from build123d import *

# Parameters (mm, degrees)
BOSS_EXTRUDE1_DEPTH      = 1040
BOSS_EXTRUDE1_DEPTH_BACK = 360
SKETCH2_R                = 7.5
BOSS_EXTRUDE2_DEPTH      = 680
SKETCH4_W                = 580
SKETCH4_H                = 10
CUT_EXTRUDE1_DEPTH       = 1252.319303775
CUT_EXTRUDE2_DEPTH       = 1252.319303775
CUT_EXTRUDE2_DEPTH_BACK  = 1252.319303775
SKETCH5_W                = 580
SKETCH5_H                = 50
CUT_EXTRUDE3_DEPTH       = 1252.319303775
CUT_EXTRUDE3_DEPTH_BACK  = 1252.319303775
SKETCH6_R                = 7.5
SKETCH8_W                = 25
SKETCH8_H                = 32
BOSS_EXTRUDE4_DEPTH      = 37.5
SKETCH9_W                = 16.002
SKETCH9_H                = 32.5
CUT_EXTRUDE4_DEPTH       = 66.8
SKETCH11_W               = 16.002
SKETCH11_H               = 64
CUT_EXTRUDE5_DEPTH       = 24
SKETCH13_R               = 2.5908
CUT_EXTRUDE6_DEPTH       = 20


with BuildPart() as part:
    # Sketch1 → Boss-Extrude1 (new, two sides: drawn at the far end of the back side and taken through both)
    with BuildSketch(Plane.XY.offset(-BOSS_EXTRUDE1_DEPTH_BACK)):
        with BuildLine():
            Line((0, 0), (-598.236730193, 0))
            ThreePointArc((-598.236730193, 0), (-599.97321197, 0.15192247), (-601.656931626, 0.603073792))
            Line((-601.656931626, 0.603073792), (-690, 32.757321084))
            Line((-690, 32.757321084), (-690, -30))
            Line((-690, -30), (-656.445665216, -30))
            Line((-656.445665216, -30), (-26.446144718, -30))
            Line((-26.446144718, -30), (0, -30))
            Line((0, -30), (0, -20.000479502))
            Line((0, -20.000479502), (0, 0))
        make_face()
    extrude(amount=BOSS_EXTRUDE1_DEPTH + BOSS_EXTRUDE1_DEPTH_BACK)

    # Sketch2 → Boss-Extrude2 (add)
    # profile 1 of 2: a face of its own
    with BuildSketch(Plane.XY):
        with BuildLine():
            Line((-690, -30), (-690, -80))
            ThreePointArc((-690, -80), (-687.071067812, -87.071067812), (-680, -90))
            Line((-680, -90), (-350, -90))
            ThreePointArc((-350, -90), (-342.928932188, -87.071067812), (-340, -80))
            Line((-340, -80), (-340, -30))
            Line((-340, -30), (-690, -30))
        make_face()
        with BuildLine():
            Line((-677.5, -72.5), (-352.5, -72.5))
            ThreePointArc((-352.5, -72.5), (-345, -80), (-352.5, -87.5))
            Line((-352.5, -87.5), (-677.5, -87.5))
            ThreePointArc((-677.5, -87.5), (-685, -80), (-677.5, -72.5))
        make_face(mode=Mode.SUBTRACT)
    # profile 2 of 2: a face of its own
    with BuildSketch(Plane.XY):
        with BuildLine():
            Line((-15, -30), (-15, -80))
            ThreePointArc((-15, -80), (-17.928932188, -87.071067812), (-25, -90))
            Line((-25, -90), (-30, -90))
            ThreePointArc((-30, -90), (-37.071067812, -87.071067812), (-40, -80))
            Line((-40, -80), (-40, -30))
            Line((-40, -30), (-15, -30))
        make_face()
        with Locations((-27.5, -80)):
            Circle(SKETCH2_R, mode=Mode.SUBTRACT)
    extrude(amount=BOSS_EXTRUDE2_DEPTH)

    # Sketch4 → Cut-Extrude1 (cut, through all)
    with BuildSketch(Plane(origin=(0, 0, 0), x_dir=(0, 0, -1), z_dir=(1, 0, 0))):
        with Locations((-340, -85)):
            Rectangle(SKETCH4_W, SKETCH4_H)
    extrude(amount=-CUT_EXTRUDE1_DEPTH, mode=Mode.SUBTRACT)

    # Sketch5 → Cut-Extrude2 (cut, two sides: drawn at the far end of the back side and taken through both)
    with BuildSketch(Plane.ZY.offset(690).offset(-CUT_EXTRUDE2_DEPTH_BACK)):
        with Locations((340, -55)):
            Rectangle(SKETCH5_W, SKETCH5_H)
    extrude(amount=CUT_EXTRUDE2_DEPTH + CUT_EXTRUDE2_DEPTH_BACK, mode=Mode.SUBTRACT)

    # Sketch6 → Cut-Extrude3 (cut, two sides: drawn at the far end of the back side and taken through both)
    with BuildSketch(Plane(origin=(0, 0, 0), x_dir=(1, 0, 0), z_dir=(0, 1, 0)).offset(-CUT_EXTRUDE3_DEPTH_BACK)):
        with Locations((-298.236730193, 60)):
            Circle(SKETCH6_R)
    extrude(amount=CUT_EXTRUDE3_DEPTH + CUT_EXTRUDE3_DEPTH_BACK, mode=Mode.SUBTRACT)

    # Sketch8 → Boss-Extrude4 (add)
    with BuildSketch(Plane.XZ.offset(30)):
        with Locations((-298.236730193, -60)):
            Rectangle(SKETCH8_W, SKETCH8_H)
    extrude(amount=BOSS_EXTRUDE4_DEPTH)

    # Sketch9 → Cut-Extrude4 (cut)
    with BuildSketch(Plane.XY.offset(-44)):
        with Locations((-298.237730193, -46.25)):
            Rectangle(SKETCH9_W, SKETCH9_H)
    extrude(amount=-CUT_EXTRUDE4_DEPTH, mode=Mode.SUBTRACT)

    # Sketch11 → Cut-Extrude5 (cut)
    with BuildSketch(Plane.XZ.offset(30)):
        with Locations((-298.237730193, -60)):
            Rectangle(SKETCH11_W, SKETCH11_H)
    extrude(amount=-CUT_EXTRUDE5_DEPTH, mode=Mode.SUBTRACT)

    # Sketch13 → Cut-Extrude6 (cut)
    with BuildSketch(Plane(origin=(0, 0, 0), x_dir=(1, 0, 0), z_dir=(0, 1, 0))):
        with Locations(Location((-300, -1015, 0), (0, 0, 180))):
            Circle(SKETCH13_R)
        with Locations(Location((-287.3, -360.9, 0), (0, 0, 180))):
            Circle(SKETCH13_R)
        with Locations(Location((-312.7, -360.9, 0), (0, 0, 180))):
            Circle(SKETCH13_R)
    extrude(amount=-CUT_EXTRUDE6_DEPTH, mode=Mode.SUBTRACT)


solid = part.part
Source: CAD feature listing. Evaluate the final solid. Frame: model axes, mm. A direction names the side the tool comes from. Round coordinates to 2 decimals unless told otherwise and drop trailing zeros. Loops run counter-clockwise (first coordinate to the right, second up) from the corner with the lowest first, then second, coordinate; pieces in that order, holes last. Notation, with made-up numbers: M 66.25,86.25 L 72.25,86.25 A16 ccw 72.25,114.25 Z; hole C 33,31 d10. An arc over 180 degrees is marked long. Return JSON: item names as keys, results as strings. Group by question number.
1. Reachability of faces 4 (the face through (-27, -53, 0)), 5 (the face through (-27, -60, 630)), 6 (the face through (-290, -48, -44)), 7 (the face through (-340, -55, 25)), 8 (the face through (-306.239, -28, -60)) from +Z, -Z, +X, -X, +Y, -Y: full face, straight path, thin tool, end or side. Return the list, or none.
2. Mould query, pull axis X, two halves, no side actions, for faces 1 (the face through (-295, 0, 330)), 2 (the face through (-513, -87.5, 655)), 3 (the face through (-285.737, -48, -60)). Classes: released by +X, released by -X, zero draft, split by the parting line, or undercut.
3. Material intervals for line 1 along X through (y, z) = (-4.5, 360.9); line 2 along Z through (x, y) = (-300, -15); line 3 along X through (y, z) = (-80, 13), sorted ascending. Write a range as from..to.
4. Section query B-B on z = 662. Output: boundary loops of the cut face in (x, y), and give its area (3 significant figures).
5. Pin query (flat end, axial travel): pin 1 (5 mm diameter, centred on x = -111.5, z = 163, fed in from -Y); pin 2 (7.5 mm diameter, centred on x = -26, y = -56.5, fed in from -Z); pin 3 (25 mm diameter, centred on x = -552, z = 663, fed in from +Y). Return the tip coordinate at first contact, or that it passes through.
6. Section query C-C on x = -441. Output: boundary loops of the cut face in (y, z).
7. Section query D-D on z = 480. Output: boundary loops of the cut face in (x, y).
8. Section query A-A on y = -46.5. Output: boundary loops of the cut face in (x, z), and give its area (3 significant figures).
Checks:
{
 "1": {"face 4": "-Z, +X, -X, -Y", "face 5": "+X, -X, -Y", "face 6": "+Z, +X, -X, -Y", "face 7": "+Z, -Z, -Y", "face 8": "none"},
 "2": {"face 1": "zero draft", "face 2": "undercut", "face 3": "released by +X"},
 "3": {"line 1": "x = -690..-315.29, -310.11..-289.89, -284.71..0", "line 2": "z = -360..-92, -28..1012.41, 1017.59..1040", "line 3": "x = -690..-685, -345..-340, -40..-35, -20..-15"},
 "4": {"outline": "M -690,-80 A10 ccw -680,-90 L -350,-90 A10 ccw -340,-80 L -340,-30 L -40,-30 L -40,-80 A10 ccw -30,-90 L -25,-90 A10 ccw -15,-80 L -15,-30 L 0,-30 L 0,0 L -598.24,0 A10 cw -601.66,0.6 L -690,32.76 Z; hole M -677.5,-87.5 L -352.5,-87.5 A7.5 ccw -352.5,-72.5 L -677.5,-72.5 A7.5 ccw Z; hole C -27.5,-80 d15", "area": "39,400 mm²"},
 "5": {"pin 1": "stops at y = -30", "pin 2": "stops at z = 0", "pin 3": "stops at y = 0"},
 "6": {"outline": "M -90,0 L -87.5,0 L -87.5,50 L -90,50 Z; M -90,630 L -87.5,630 L -87.5,680 L -90,680 Z; M -72.5,0 L -30,0 L -30,-360 L 0,-360 L 0,1040 L -30,1040 L -30,680 L -72.5,680 L -72.5,630 L -30,630 L -30,50 L -72.5,50 Z"},
 "7": {"outline": "M -690,-30 L 0,-30 L 0,0 L -598.24,0 A10 cw -601.66,0.6 L -690,32.76 Z"},
 "8": {"outline": "M -690,0 L -340,0 L -340,50 L -690,50 Z; M -690,630 L -340,630 L -340,680 L -690,680 Z; M -310.74,-76 L -306.24,-76 L -306.24,-44 L -310.74,-44 Z; M -290.24,-76 L -285.74,-76 L -285.74,-44 L -290.24,-44 Z; M -40,0 L -15,0 L -15,50 L -40,50 Z; M -40,630 L -15,630 L -15,680 L -40,680 Z", "area": "37,800 mm²"}
}
